```python
from build123d import *

# Parameters (mm, degrees)
BOSS_EXTRUDE1_START     = -5
BOSS_EXTRUDE1_OUTLINE_R = 1.925
BOSS_EXTRUDE1_DEPTH     = 5
SKETCH4_R               = 1.6
CUT_EXTRUDE2_DEPTH      = 161.661912101
FILLET1_R               = 15
SKETCH5_R               = 2.1
SKETCH5_R_2             = 2.6
CUT_EXTRUDE4_DEPTH      = 161.661912218
SKETCH6_W               = 233.09675901
SKETCH6_H               = 87.107773224
CUT_EXTRUDE5_DEPTH      = 2


with BuildPart() as part:
    # Boss-Extrude1: read off the stored shape, not the designer's step
    # Boss-Extrude1 outline → Boss-Extrude1 (new body)
    with BuildSketch(Plane.XY.offset(5).offset(BOSS_EXTRUDE1_START)):
        with BuildLine():
            ThreePointArc((149.353851183, 10.916367847), (81.584978704, 16.866619507), (13.564040933, 17.951790818))
            ThreePointArc((13.564040933, 17.951790818), (-22.408339146, -2.028875729), (16.567779435, -15.223622585))
            ThreePointArc((16.567779435, -15.223622585), (81.747231754, -9.530296146), (147.159069574, -10.96780908))
            ThreePointArc((147.159069574, -10.96780908), (158.945093507, -1.097692183), (149.353851183, 10.916367847))
        make_face()
        with Locations((40, 2.5)):
            Circle(BOSS_EXTRUDE1_OUTLINE_R, mode=Mode.SUBTRACT)
        with Locations((95, 2.5)):
            Circle(BOSS_EXTRUDE1_OUTLINE_R, mode=Mode.SUBTRACT)
    extrude(amount=BOSS_EXTRUDE1_DEPTH)

    # Sketch4 → Cut-Extrude2 (cut, through all)
    with BuildSketch(Plane.XY.offset(5)):
        with Locations((0, 17)):
            Circle(SKETCH4_R)
        with Locations((16.167960777, 5.253288904)):
            Circle(SKETCH4_R)
        with Locations((9.992349289, -13.753288904)):
            Circle(SKETCH4_R)
        with Locations((-9.992349289, -13.753288904)):
            Circle(SKETCH4_R)
        with Locations((-16.167960777, 5.253288904)):
            Circle(SKETCH4_R)
    extrude(amount=-CUT_EXTRUDE2_DEPTH, mode=Mode.SUBTRACT)

    # Fillet1
    fillet1_edges = [part.edges().sort_by_distance(p)[0] for p in [
        (16.567779435, -15.223622585, 2.5),
        (13.564040933, 17.951790818, 2.5),
    ]]
    fillet(fillet1_edges, radius=FILLET1_R)

    # Sketch5 → Cut-Extrude4 (cut, through all)
    with BuildSketch(Plane.XY.offset(5)):
        Circle(SKETCH5_R)
        with Locations((148, 0)):
            Circle(SKETCH5_R_2)
        with Locations((95, 2.5)):
            Circle(SKETCH5_R_2)
        with Locations((40, 2.5)):
            Circle(SKETCH5_R_2)
    extrude(amount=-CUT_EXTRUDE4_DEPTH, mode=Mode.SUBTRACT)

    # Sketch6 → Cut-Extrude5 (cut)
    with BuildSketch(Plane.XY.offset(5)):
        with Locations((68.481602645, 0)):
            Rectangle(SKETCH6_W, SKETCH6_H)
    extrude(amount=-CUT_EXTRUDE5_DEPTH, mode=Mode.SUBTRACT)


solid = part.part
```
Geometry check sheet. Reference: the model listing, model coordinates, mm. Round coordinates to 2 decimals unless told otherwise and drop trailing zeros. Loops run counter-clockwise (first coordinate to the right, second up) from the corner with the lowest first, then second, coordinate; pieces in that order, holes last. Notation, with made-up numbers: (38, 42) - (87, 42) arc R23 cw to (87, 79) - close; hole circle Ø10 at (-39, -5). An arc over 180 degrees is marked (long way). Write each question's results on one line, items separated by ' | '. Start each with the question number.
Q1. Cross-section at D-D on z = 0.6. State how many separate pieces and enclosed holes the cut face has, and give its area (3 significant figures).
Q2. Thickness scan on line 1 (Y direction, x = 0, z = 1.55); line 2 (X direction, y = 3.5, z = 0.25); line 3 (Y direction, x = 94, z = 0.5). Record the ranges inside material, lowest first. Write a range as [from, to].
Q3. Cross-section at A-A on x = 0. Enter the section's corners in (y, z), and give its area (3 significant figures).
Q4. Cross-section at B-B on x = 40. Enter the section's corners in (y, z).
Q5. Cross-section at C-C on x = 95. Enter the section's corners in (y, z), and give its area (3 significant figures).
Q6. Gauge pin test, flat ends, axial feed: P1, Ø5, axis at x = 3, y = 7, coming from the -Z side; P2, Ø1, axis at x = 38, z = 1.5, coming from the -Y side. Record the tip position at first contact, or that the pin passes through.
Q7. Release check for a two-part mould opening along X. For faces 1 (the cylindrical face through (92.4, 2.6, 1.5)), 2 (the flat face through (47, 0, 0)), 3 (the cylindrical face through (-22.463, -1.284, 1.479)) record: +X half, -X half, draft (parallel to the pull), parting line (faces both ways), or undercut.
Answers below:
1) separate pieces: 1 | enclosed holes: 9 | area: 5,070 mm²
2) line 1: y = [-22.5, -2.1], [2.1, 15.4], [18.6, 22.5] | line 2: x = [-22.23, 37.6], [42.4, 92.6], [97.4, 158.43] | line 3: y = [-9.26, 0.1], [4.9, 16.14]
3) outline: (-22.5, 0) - (-2.1, 0) - (-2.1, 3) - (-22.5, 3) - close; (2.1, 0) - (15.4, 0) - (15.4, 3) - (2.1, 3) - close; (18.6, 0) - (22.5, 0) - (22.5, 3) - (18.6, 3) - close | area: 113 mm²
4) outline: (-12.35, 0) - (-0.1, 0) - (-0.1, 3) - (-12.35, 3) - close; (5.1, 0) - (18.11, 0) - (18.11, 3) - (5.1, 3) - close
5) outline: (-9.24, 0) - (-0.1, 0) - (-0.1, 3) - (-9.24, 3) - close; (5.1, 0) - (16.08, 0) - (16.08, 3) - (5.1, 3) - close | area: 60.4 mm²
6) P1: stops at z = 0 | P2: stops at y = -12.61
7) face 1: undercut | face 2: draft | face 3: parting line
